from build123d import *

# Parameters (mm, degrees)
SKETCH1_W           = 190.5
SKETCH1_H           = 190.5
SKETCH1_R           = 1.905
SKETCH1_R_2         = 1.778
BOSS_EXTRUDE1_DEPTH = 6.35
SKETCH2_W           = 54.8
SKETCH2_H           = 54.8
CUT_EXTRUDE4_DEPTH  = 10
SKETCH4_R           = 1.5875
CUT_EXTRUDE5_DEPTH  = 10
SKETCH5_R           = 3.175
CUT_EXTRUDE6_DEPTH  = 7.35


with BuildPart() as part:
    # Sketch1 → Boss-Extrude1 (new body)
    with BuildSketch(Plane(origin=(0, 0, 0), x_dir=(1, 0, 0), z_dir=(0, 1, 0))):
        Rectangle(SKETCH1_W, SKETCH1_H)
        with Locations((-11.303, 11.303)):
            Circle(SKETCH1_R, mode=Mode.SUBTRACT)
        with Locations((-11.303, -11.303)):
            Circle(SKETCH1_R, mode=Mode.SUBTRACT)
        with Locations((11.303, 11.303)):
            Circle(SKETCH1_R, mode=Mode.SUBTRACT)
        with Locations((11.303, -11.303)):
            Circle(SKETCH1_R, mode=Mode.SUBTRACT)
        with Locations((-78.9, 86.55)):
            Circle(SKETCH1_R_2, mode=Mode.SUBTRACT)
        with Locations((-91.6, 86.55)):
            Circle(SKETCH1_R_2, mode=Mode.SUBTRACT)
        with Locations((91.6, -86.55)):
            Circle(SKETCH1_R_2, mode=Mode.SUBTRACT)
        with Locations((78.9, -86.55)):
            Circle(SKETCH1_R_2, mode=Mode.SUBTRACT)
        with Locations((-86.55, -78.9)):
            Circle(SKETCH1_R_2, mode=Mode.SUBTRACT)
        with Locations((-86.55, -91.6)):
            Circle(SKETCH1_R_2, mode=Mode.SUBTRACT)
    extrude(amount=BOSS_EXTRUDE1_DEPTH)

    # Sketch2 → Cut-Extrude4 (cut)
    with BuildSketch(Plane.XZ):
        Rectangle(SKETCH2_W, SKETCH2_H)
    extrude(amount=-CUT_EXTRUDE4_DEPTH, mode=Mode.SUBTRACT)

    # Sketch4 → Cut-Extrude5 (cut)
    with BuildSketch(Plane.XZ):
        with Locations((-31.75, 31.75)):
            Circle(SKETCH4_R)
        with Locations((31.75, 31.75)):
            Circle(SKETCH4_R)
        with Locations((31.75, -31.75)):
            Circle(SKETCH4_R)
        with Locations((-31.75, -31.75)):
            Circle(SKETCH4_R)
    extrude(amount=-CUT_EXTRUDE5_DEPTH, mode=Mode.SUBTRACT)

    # Sketch5 → Cut-Extrude6 (cut, through all)
    with BuildSketch(Plane.XZ):
        with Locations((76.33, -76.33)):
            Circle(SKETCH5_R)
        with Locations((76.33, 76.33)):
            Circle(SKETCH5_R)
        with Locations((-76.33, -76.33)):
            Circle(SKETCH5_R)
        with Locations((-76.33, 76.33)):
            Circle(SKETCH5_R)
    extrude(amount=-CUT_EXTRUDE6_DEPTH, mode=Mode.SUBTRACT)


solid = part.part
Geometry: final body of the model. Coordinates: model frame, mm. A direction names the side the tool comes from. Give positions to 0.01 mm unless a question says otherwise; leave off trailing zeros. Loops run counter-clockwise (first coordinate to the right, second up) from the corner with the lowest first, then second, coordinate; pieces in that order, holes last. Notation, with made-up numbers: (18.25, -25.5) -> (23.25, -25.5) arc R17 cw to (23.25, -21.5) -> close; hole circle Ø11 at (-27, 56). An arc over 180 degrees is marked (long way). Put each result on its own line as item: value.
1. Set-up query: faces 1 (the flat face through (0, 3, 27.4)), 2 (the flat face through (41, 6.35, -1)). Return all of +Z, -Z, +X, -X, +Y, -Y with unobstructed straight access to the full face (end or side cutting, diameter ignored); none if empty.
Taken from the geometry:
face 1: +Y, -Y
face 2: +Z, -Z, +X, -X, +Y
2. Ray query, line 1 along X through (y, z) = (4.75, -86.55); line 2 along Z through (x, y) = (31.75, 2.5); line 3 along Z through (x, y) = (-76.33, 3.5) (3 decimals). Return the intervals inside material, ascending. Write a range as [from, to].
Taken from the geometry:
line 1: x = [-95.25, -93.38], [-89.82, -80.68], [-77.12, 95.25]
line 2: z = [-95.25, -33.34], [-30.16, 30.16], [33.34, 95.25]
line 3: z = [-95.25, -79.505], [-73.155, 73.155], [79.505, 95.25]
3. Cut plane B-B (x = 0). Return the cut outline in (y, z).
Taken from the geometry:
outline: (0, -95.25) -> (6.35, -95.25) -> (6.35, -27.4) -> (0, -27.4) -> close; (0, 27.4) -> (6.35, 27.4) -> (6.35, 95.25) -> (0, 95.25) -> close
4. Cut plane C-C (y = 2.5). Count the separate pieces of the cut face and the enclosed holes in it, plus the area to 3 significant figures.
Taken from the geometry:
separate pieces: 1
enclosed holes: 15
area: 33,100 mm2
5. Pull-direction query (X, two-part tool) for faces 3 (the cylindrical face through (-74.623, 3.131, 79.007)), 4 (the flat face through (-95.25, 3, 1)), 5 (the flat face through (-1, 3, 95.25)); classes: released by +X, released by -X, zero draft, split by the parting line, or undercut.
Taken from the geometry:
face 3: undercut
face 4: released by -X
face 5: zero draft
6. Pin query (flat end, axial travel): P1, Ø5.5, axis at x = -91.6, z = -86.55, coming from the +Y side; P2, Ø2, axis at x = 9.5, z = 25, coming from the +Y side. Return the tip coordinate at first contact, or that it passes through.
Taken from the geometry:
P1: stops at y = 6.35
P2: passes through
7. Cut plane A-A (z = 23.5). Return the cut outline in (x, y).
Taken from the geometry:
outline: (-95.25, 0) -> (-27.4, 0) -> (-27.4, 6.35) -> (-95.25, 6.35) -> close; (27.4, 0) -> (95.25, 0) -> (95.25, 6.35) -> (27.4, 6.35) -> close
